Study the drawing (mm; zero at the part's minimum x, y, z) and answer. A direction names the side the tool comes from. Round coordinates to 2 decimals unless told otherwise and drop trailing zeros. Loops run counter-clockwise (first coordinate to the right, second up) from the corner with the lowest first, then second, coordinate; pieces in that order, holes last. Notation, with made-up numbers: (-34.75, 21.25) -> (-22.75, 21.25) arc R14 cw to (-22.75, 36.25) -> close; hole circle Ø4 at (70, -28.5). An arc over 180 degrees is marked (long way). Answer in a Markdown table with one row per item. Add a question column.
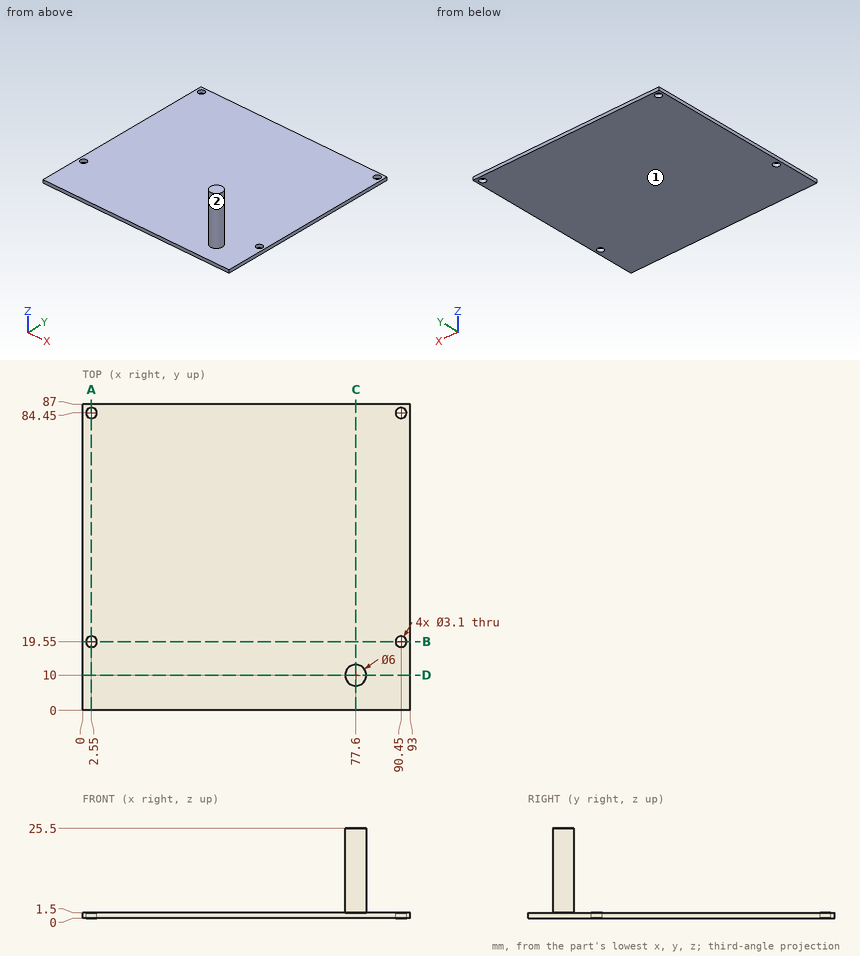
Item 1: Section A-A, the plane x = 2.55 is taken. Write down the section's boundary in (y, z), and give its area (3 significant figures).
Item 2: Section D-D, the plane y = 10 is taken. Write down the section's boundary in (x, z).
Item 3: Section B-B, the plane y = 19.55 is taken. Write down the section's boundary in (x, z).
Item 4: Section C-C, the plane x = 77.6 is taken. Write down the section's boundary in (y, z).
Item 5: Flat-ended cylindrical pins translate along their axes: P1, Ø1.9, axis at x = 2.55, y = 84.45, coming from the -Z side; P2, Ø6, axis at x = 72.5, y = 25, coming from the +Z side; P3, Ø4, axis at x = 90.45, y = 19.55, coming from the -Z side; P4, Ø1, axis at x = 74.5, z = 16.5, coming from the -Y side. Find the tip coordinate at first contact, or state that the pin passes through.
Item 6: For the marked faces 1 and 2, determine the directions among +Z, -Z, +X, -X, +Y, -Y from which every point of the face is accessible in a straight line to the end or side of a thin tool.
Item 7: Consider L1, parallel to X at y = 84.45, z = 0.4; L2, parallel to Y at x = 2.55, z = 0.85; L3, parallel to Z at x = 13.5, y = 48. Determine where each line is inside the solid, lowest interval first. Write a range as from..to.
Here are the results:
| question | item | result |
|---|---|---|
| 1 | outline | (0, 0) -> (18, 0) -> (18, 1.5) -> (0, 1.5) -> close; (21.1, 0) -> (82.9, 0) -> (82.9, 1.5) -> (21.1, 1.5) -> close; (86, 0) -> (87, 0) -> (87, 1.5) -> (86, 1.5) -> close |
| 1 | area | 121 mm² |
| 2 | outline | (0, 0) -> (93, 0) -> (93, 1.5) -> (80.6, 1.5) -> (80.6, 25.5) -> (74.6, 25.5) -> (74.6, 1.5) -> (0, 1.5) -> close |
| 3 | outline | (0, 0) -> (1, 0) -> (1, 1.5) -> (0, 1.5) -> close; (4.1, 0) -> (88.9, 0) -> (88.9, 1.5) -> (4.1, 1.5) -> close; (92, 0) -> (93, 0) -> (93, 1.5) -> (92, 1.5) -> close |
| 4 | outline | (0, 0) -> (87, 0) -> (87, 1.5) -> (13, 1.5) -> (13, 25.5) -> (7, 25.5) -> (7, 1.5) -> (0, 1.5) -> close |
| 5 | P1 | passes through |
| 5 | P2 | stops at z = 1.5 |
| 5 | P3 | stops at z = 0 |
| 5 | P4 | stops at y = 8.5 |
| 6 | face 1 | -Z, +X, -X, +Y, -Y |
| 6 | face 2 | +Z |
| 7 | L1 | x = 0..1, 4.1..88.9, 92..93 |
| 7 | L2 | y = 0..18, 21.1..82.9, 86..87 |
| 7 | L3 | z = 0..1.5 |
